Work out the finished part from the listing and answer in its coordinate system (mm). A direction names the side the tool comes from. Give positions to 0.01 mm unless a question says otherwise; leave off trailing zeros. Order: outer loops, then holes, each group sorted by start corner. A loop starts at its lowest first (then second) coordinate and runs counter-clockwise, first axis right, second up. Notation, with made-up numbers: M 78,-20.75 L 84,-20.75 A9 ccw 84,-14.75 Z; hole C 73,5 d9. An arc over 180 degrees is marked long. One line per item, written item: value.
from build123d import *

# Parameters (mm, degrees)
SKETCH1_R               = 9.5
SKETCH1_R_2             = 6.35
BOSS_EXTRUDE1_DEPTH     = 13.25
SKETCH2_W               = 73.338944958
SKETCH2_H               = 12.5
CUT_EXTRUDE3_DEPTH      = 38
CUT_EXTRUDE5_DEPTH      = 124.21282036
CUT_EXTRUDE5_DEPTH_BACK = 6
CUT_EXTRUDE6_DEPTH      = 124.21282036
CUT_EXTRUDE6_DEPTH_BACK = 6
CUT_EXTRUDE8_DEPTH      = 5
CUT_EXTRUDE8_DRAFT      = -2
MIRROR8_COPY_1_DEPTH    = 5
MIRROR8_COPY_1_DRAFT    = -2


with BuildPart() as part:
    # Sketch1 → Boss-Extrude1 (new, symmetric)
    with BuildSketch(Plane(origin=(0, 0, 0), x_dir=(1, 0, 0), z_dir=(0, 1, 0))):
        with BuildLine():
            Line((0, 0), (-62, 0))
            ThreePointArc((-62, 0), (-75.125587601, 4.90964049), (-81.806983567, 17.228104986))
            Line((-81.806983567, 17.228104986), (-88.547021707, 65.390038979))
            ThreePointArc((-88.547021707, 65.390038979), (-78.78369233, 80.716074763), (-62.110282709, 73.49060696))
            ThreePointArc((-62.110282709, 73.49060696), (-36.56849942, 45.611382856), (0, 36))
            Line((0, 36), (0, 26.5))
            Line((0, 26.5), (-22, 26.5))
            ThreePointArc((-22, 26.5), (-28.5, 20), (-22, 13.5))
            Line((-22, 13.5), (0, 13.5))
            Line((0, 13.5), (0, 0))
        make_face()
        with Locations(Location((-62, 20, 0), (0, 0, 270))):
            Circle(SKETCH1_R, mode=Mode.SUBTRACT)
        with Locations(Location((-74.68213321, 67.330365488, 0), (0, 0, 270))):
            Circle(SKETCH1_R_2, mode=Mode.SUBTRACT)
    extrude(amount=BOSS_EXTRUDE1_DEPTH, both=True)

    # Sketch2 → Cut-Extrude3 (cut)
    with BuildSketch(Plane(origin=(0, 0, 0), x_dir=(0, 0, -1), z_dir=(1, 0, 0))):
        with Locations((36.669472479, 0)):
            Rectangle(SKETCH2_W, SKETCH2_H)
    extrude(amount=-CUT_EXTRUDE3_DEPTH, mode=Mode.SUBTRACT)

    # Sketch3 → Cut-Extrude5 (cut, two sides: drawn at the far end of the back side and taken through both)
    with BuildSketch(Plane(origin=(0, 13.25, 0), x_dir=(1, 0, 0), z_dir=(0, 1, 0)).offset(-CUT_EXTRUDE5_DEPTH_BACK)):
        with BuildLine():
            Line((-251.132551902, 188.14493361), (-86.7667399, 52.668773448))
            ThreePointArc((-86.7667399, 52.668773448), (-71.019379836, 48.686754311), (-57.948932679, 58.330365488))
            Line((-57.948932679, 58.330365488), (-51.906439966, 58.330365488))
            Line((-51.906439966, 58.330365488), (161.095696471, 58.330365488))
            Line((161.095696471, 58.330365488), (289.053745356, 464.663207174))
            Line((289.053745356, 464.663207174), (-123.174503017, 594.477775296))
            Line((-123.174503017, 594.477775296), (-251.132551902, 188.14493361))
        make_face()
    extrude(amount=CUT_EXTRUDE5_DEPTH + CUT_EXTRUDE5_DEPTH_BACK, mode=Mode.SUBTRACT)

    # Sketch4 → Cut-Extrude6 (cut, two sides: drawn at the far end of the back side and taken through both)
    with BuildSketch(Plane.XZ.offset(13.25).offset(-CUT_EXTRUDE6_DEPTH_BACK)):
        with BuildLine():
            Line((-251.132551902, -188.14493361), (-86.7667399, -52.668773448))
            ThreePointArc((-86.7667399, -52.668773448), (-71.019379836, -48.686754311), (-57.948932679, -58.330365488))
            Line((-57.948932679, -58.330365488), (-51.906439966, -58.330365488))
            Line((-51.906439966, -58.330365488), (161.095696471, -58.330365488))
            Line((161.095696471, -58.330365488), (289.053745356, -464.663207174))
            Line((289.053745356, -464.663207174), (-123.174503017, -594.477775296))
            Line((-123.174503017, -594.477775296), (-251.132551902, -188.14493361))
        make_face()
    extrude(amount=CUT_EXTRUDE6_DEPTH + CUT_EXTRUDE6_DEPTH_BACK, mode=Mode.SUBTRACT)


with BuildPart() as cut_extrude8_tool:
    # Sketch6 → Cut-Extrude8 (with draft: the straight prism first)
    with BuildSketch(Plane(origin=(0, 13.25, 0), x_dir=(1, 0, 0), z_dir=(0, 1, 0))):
        with BuildLine():
            Line((-2, 28.5), (-2, 33.971784495))
            ThreePointArc((-2, 33.971784495), (-29.743751646, 39.819333442), (-52.793597737, 56.330365488))
            Line((-52.793597737, 56.330365488), (-56.79358939, 56.330365488))
            ThreePointArc((-56.79358939, 56.330365488), (-68.976857381, 47.120223784), (-84.177824667, 48.599859789))
            Line((-84.177824667, 48.599859789), (-79.826285211, 17.505294488))
            ThreePointArc((-79.826285211, 17.505294488), (-73.813028841, 6.418676441), (-62, 2))
            Line((-62, 2), (-2, 2))
            Line((-2, 2), (-2, 11.5))
            Line((-2, 11.5), (-22, 11.5))
            ThreePointArc((-22, 11.5), (-30.5, 20), (-22, 28.5))
            Line((-22, 28.5), (-2, 28.5))
        make_face()
    extrude(amount=-CUT_EXTRUDE8_DEPTH)
    # Cut-Extrude8: the draft: its side faces are tilted about the plane it starts from
    cut_extrude8_sides = [cut_extrude8_tool.faces().sort_by_distance(p)[0] for p in [
        (-12, 10.75, -28.5),
        (-2, 10.75, -31.235892247),
        (-29.743751646, 10.75, -39.819333442),
        (-54.793593564, 10.75, -56.330365488),
        (-68.976857381, 10.75, -47.120223784),
        (-82.002054939, 10.75, -33.052577138),
        (-73.813028841, 10.75, -6.418676441),
        (-32, 10.75, -2),
        (-2, 10.75, -6.75),
        (-12, 10.75, -11.5),
        (-30.5, 10.75, -20),
    ]]
    draft(cut_extrude8_sides, Plane(origin=(0, 13.25, 0), x_dir=(1, 0, 0), z_dir=(0, 1, 0)), CUT_EXTRUDE8_DRAFT)


with BuildPart() as part_1:
    add(part.part)

    # Cut-Extrude8: cut by cut_extrude8_tool
    add(cut_extrude8_tool.part, mode=Mode.SUBTRACT)


with BuildPart() as mirror8_copy_1_tool:
    # Mirror8 copy 1 sketch → Mirror8 copy 1 (with draft: the straight prism first)
    with BuildSketch(Plane.XZ.offset(13.25)):
        with BuildLine():
            Line((-2, -28.5), (-2, -33.971784495))
            ThreePointArc((-2, -33.971784495), (-29.743751646, -39.819333442), (-52.793597737, -56.330365488))
            Line((-52.793597737, -56.330365488), (-56.79358939, -56.330365488))
            ThreePointArc((-56.79358939, -56.330365488), (-68.976857381, -47.120223784), (-84.177824667, -48.599859789))
            Line((-84.177824667, -48.599859789), (-79.826285211, -17.505294488))
            ThreePointArc((-79.826285211, -17.505294488), (-73.813028841, -6.418676441), (-62, -2))
            Line((-62, -2), (-2, -2))
            Line((-2, -2), (-2, -11.5))
            Line((-2, -11.5), (-22, -11.5))
            ThreePointArc((-22, -11.5), (-30.5, -20), (-22, -28.5))
            Line((-22, -28.5), (-2, -28.5))
        make_face()
    extrude(amount=-MIRROR8_COPY_1_DEPTH)
    # Mirror8 copy 1: the draft: its side faces are tilted about the plane it starts from
    mirror8_copy_1_sides = [mirror8_copy_1_tool.faces().sort_by_distance(p)[0] for p in [
        (-12, -10.75, -28.5),
        (-2, -10.75, -31.235892247),
        (-29.743751646, -10.75, -39.819333442),
        (-54.793593564, -10.75, -56.330365488),
        (-68.976857381, -10.75, -47.120223784),
        (-82.002054939, -10.75, -33.052577138),
        (-73.813028841, -10.75, -6.418676441),
        (-32, -10.75, -2),
        (-2, -10.75, -6.75),
        (-12, -10.75, -11.5),
        (-30.5, -10.75, -20),
    ]]
    draft(mirror8_copy_1_sides, Plane.XZ.offset(13.25), MIRROR8_COPY_1_DRAFT)


with BuildPart() as part_2:
    add(part_1.part)

    # Mirror8 copy 1: cut by mirror8_copy_1_tool
    add(mirror8_copy_1_tool.part, mode=Mode.SUBTRACT)


solid = part_2.part
(1) Section B-B, the plane z = -20 is taken. Give the vertices of the cut face in (x, y), then the cut area to 3 significant figures.
Findings:
outline: M -82.19,-13.25 L -80.18,-13.25 L -80,-8.25 L -71.5,-8.25 L -71.5,8.25 L -80,8.25 L -80.18,13.25 L -82.19,13.25 Z; M -52.5,-8.25 L -30.67,-8.25 L -30.5,-13.25 L -28.5,-13.25 L -28.5,-6.25 L -38,-6.25 L -38,6.25 L -28.5,6.25 L -28.5,13.25 L -30.5,13.25 L -30.67,8.25 L -52.5,8.25 Z
area: 496 mm^2
(2) Find the intervals of material crossed by probe 1 along Y at (x, z) = (-71, -54); probe 2 along Z at (x, y) = (-46, 5); probe 3 along Y at (x, z) = (-70.5, -24.5), in increasing order. Write a range as from..to.
Findings:
probe 1: y = -7.25..7.25
probe 2: z = -52.49..0
probe 3: y = -8.25..8.25
(3) Which of the six approach directions +Z, -Z, +X, -X, +Y, -Y give full straight-line access (tool end or side, diameter ignored) to faces 5 (the flat face through (-23, -6.25, -13)), 6 (the conical face through (-30.584, -10.785, -19.811)), 7 (the flat face through (-55, -10, -58.33)), 8 (the cylindrical face through (-28.5, 9.8, -20.1)), 9 (the flat face through (-85.13, 0.19, -40.97))?
Findings:
face 5: +Z, -Z, +X
face 6: -Y
face 7: -Z, +X, -X, -Y
face 8: +X, +Y, -Y
face 9: +Z, -X, +Y, -Y
(4) Given P1, Ø6.5, axis at x = -55.5, y = 9, coming from the -Z side; P2, Ø10, axis at x = -76, z = -68.5, coming from the -Y side; P3, Ø5, axis at y = -10.5, z = -47.5, coming from the -X side; P4, Ø4, axis at x = -56, z = -23.5, coming from the +Y side, each flat-ended and moving along its own axis, determine where each tip first touches the part or whether it passes through.
Findings:
P1: stops at z = -66.64
P2: stops at y = -7.25
P3: stops at x = -86.39
P4: passes through
(5) Section A-A, the plane y = 9.5 is taken. Give the vertices of the cut face in (x, z) (3 decimals).
Findings:
outline: M -86.767,-52.669 A19 cw -57.949,-58.33 L -51.906,-58.33 A67 cw 0,-36 L 0,-26.5 L -22,-26.5 A6.5 cw -22,-13.5 L 0,-13.5 L 0,0 L -62,0 A20 ccw -81.807,-17.228 Z; hole M -84.014,-48.371 A21.131 cw -56.721,-56.199 L -52.851,-56.199 A69.131 cw -2.131,-33.841 L -2.131,-28.631 L -22,-28.631 A8.631 cw -22,-11.369 L -2.131,-11.369 L -2.131,-2.131 L -62,-2.131 A17.869 ccw -79.697,-17.523 Z
(6) Determine the mould class of faces 1 (the flat face through (-23, 6.25, -13)), 2 (the flat face through (-30, -13.25, -21)), 3 (the cylindrical face through (-71.25, 10.208, -48.643)), 4 (the flat face through (-71, 7.25, -61)) for opening direction Y: pulls with the +Y half, pulls with the -Y half, needs draft (parallel to the pull), parting line crosses it, or undercut.
Findings:
face 1: undercut
face 2: pulls with the -Y half
face 3: needs draft
face 4: pulls with the +Y half
(7) Section C-C, the plane y = -4 is taken. Give the vertices of the cut face in (x, z) (3 decimals), then the cut area to 3 significant figures.
Findings:
outline: M -88.547,-65.39 A14 ccw -62.11,-73.491 A67 cw -38,-46.5 L -38,0 L -62,0 A20 ccw -81.807,-17.228 Z; hole C -74.682,-67.33 d12.7; hole C -62,-20 d19
area: 2,700 mm^2
